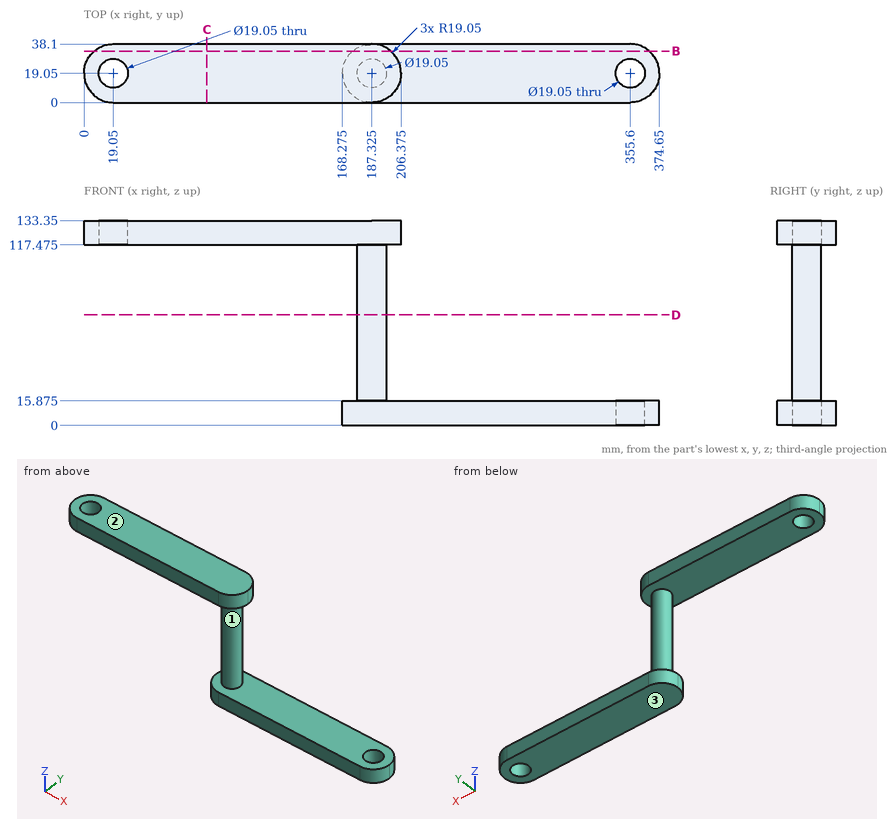
Input: dimensioned drawing with shaded views. Units: mm. Origin: part minimum x, y, z. Round coordinates to 2 decimals unless told otherwise and drop trailing zeros. Loops run counter-clockwise (first coordinate to the right, second up) from the corner with the lowest first, then second, coordinate; pieces in that order, holes last. Notation, with made-up numbers: M 85,0.5 L 121,0.5 A12 ccw 121,14.5 Z; hole C -27,87.5 d3. An arc over 180 degrees is marked long. Answer in a Markdown table with one row per item. Add a question column.
1. Section B-B (y = 33.5). Output: boundary loops of the cut face in (x, z) (3 decimals), and give its area (3 significant figures).
2. Mould query, pull axis Z, two halves, no side actions, for the marked faces 1, 2 and 3. Classes: released by +Z, released by -Z, zero draft, split by the parting line, or undercut.
3. Ray query, probe 1 along X at (y, z) = (19, 7); probe 2 along Y at (x, z) = (355, 8); probe 3 along Z at (x, y) = (170, 19) (3 decimals). Return the intervals inside material, ascending.
4. Contact query for flat-ended pins moving along their axis: pin 1 (15 mm diameter, centred on x = 355.6, y = 19.05, fed in from +Z); pin 2 (5 mm diameter, centred on y = 9.5, z = 60, fed in from +X); pin 3 (10 mm diameter, centred on x = 174, z = 83, fed in from -Y); pin 4 (1 mm diameter, centred on y = 9.5, z = 14.5, fed in from +X). Output: stop coordinate, or through.
5. Section D-D (z = 72). Output: boundary loops of the cut face in (x, y) (3 decimals), and give its area (3 significant figures).
6. Section C-C (x = 80). Output: boundary loops of the cut face in (y, z) (3 decimals).
Values follow:
| question | item | result |
|---|---|---|
| 1 | outline | M 6.636,117.475 L 199.739,117.475 L 199.739,133.35 L 6.636,133.35 Z; M 174.911,0 L 368.014,0 L 368.014,15.875 L 174.911,15.875 Z |
| 1 | area | 6,130 mm^2 |
| 2 | face 1 | undercut |
| 2 | face 2 | released by +Z |
| 2 | face 3 | released by -Z |
| 3 | probe 1 | 168.28 to 346.08, 365.12 to 374.65 |
| 3 | probe 2 | 0 to 9.54, 28.56 to 38.1 |
| 3 | probe 3 | 0 to 15.875, 117.475 to 133.35 |
| 4 | pin 1 | through |
| 4 | pin 2 | x = 193.73 |
| 4 | pin 3 | y = 14.42 |
| 4 | pin 4 | x = 372.36 |
| 5 | outline | C 187.325,19.05 d19.05 |
| 5 | area | 285 mm^2 |
| 6 | outline | M 0,117.475 L 38.1,117.475 L 38.1,133.35 L 0,133.35 Z |
